from build123d import *

# Parameters (mm, degrees)
SKETCH2_W            = 120
SKETCH2_H            = 120
BOSS_EXTRUDE1_DEPTH  = 8
SKETCH4_R            = 12.5
CUT_EXTRUDE1_DEPTH   = 86.229103011
SKETCH6_R            = 5
CUT_EXTRUDE2_DEPTH   = 86.229103011
LPATTERN1_COUNT      = 2
LPATTERN1_PITCH      = 80
LPATTERN1_COUNT_DIR2 = 2
LPATTERN1_PITCH_DIR2 = 80
FILLET2_R            = 20


with BuildPart() as part:
    # Sketch2 → Boss-Extrude1 (new body)
    with BuildSketch(Plane.XY):
        Rectangle(SKETCH2_W, SKETCH2_H)
    extrude(amount=BOSS_EXTRUDE1_DEPTH)

    # Sketch4 → Cut-Extrude1 (cut, through all)
    with BuildSketch(Plane.XY.offset(8)):
        Circle(SKETCH4_R)
    extrude(amount=-CUT_EXTRUDE1_DEPTH, mode=Mode.SUBTRACT)

    # Sketch6 → Cut-Extrude2 (cut, through all)
    with BuildSketch(Plane.XY.offset(8)):
        with Locations((-40, 40)):
            Circle(SKETCH6_R)
    cut_extrude2 = extrude(amount=-CUT_EXTRUDE2_DEPTH, mode=Mode.SUBTRACT)

    # LPattern1: Cut-Extrude2 2 × 2
    with Locations(*[(i * LPATTERN1_PITCH, -j * LPATTERN1_PITCH_DIR2, 0) for i in range(LPATTERN1_COUNT) for j in range(LPATTERN1_COUNT_DIR2) if (i, j) != (0, 0)]):
        add(cut_extrude2, mode=Mode.SUBTRACT)

    # Fillet2
    fillet2_edges = [part.edges().sort_by_distance(p)[0] for p in [
        (60, -60, 4),
        (60, 60, 4),
    ]]
    fillet(fillet2_edges, radius=FILLET2_R)


solid = part.part
CAD build for the part. Positions are in the model's coordinates, mm. Give positions to 0.01 mm unless a question says otherwise; leave off trailing zeros. Loops run counter-clockwise (first coordinate to the right, second up) from the corner with the lowest first, then second, coordinate; pieces in that order, holes last. Notation, with made-up numbers: M 40.5,-36.75 L 87.5,-36.75 A16 ccw 87.5,-12.75 Z; hole C 10.5,74.5 d8. An arc over 180 degrees is marked long. Write each question's results on one line, items separated by ' | '.
Q1. Flat gauge pins, fed straight in: P1, Ø8, axis at x = 40, y = 40, coming from the +Z side; P2, Ø1.5, axis at x = 47.5, z = 1, coming from the -Y side. Where does each tip first touch, or does it go through?
Geometry check:
P1: passes through | P2: stops at y = -58.83
Q2. Mould opens along Y. For faces 1 (the face through (-14, 1, 0)), 2 (the face through (-11, -60, 4)), 3 (the face through (-45, -40, 4)) say: pulls with the +Y half, pulls with the -Y half, needs draft (parallel to the pull), parting line crosses it, or undercut.
Geometry check:
face 1: needs draft | face 2: pulls with the -Y half | face 3: undercut
Q3. Band-saw the part on B-B on z = 1.5. Write the cut outline in (x, y).
Geometry check:
outline: M -60,-60 L 40,-60 A20 ccw 60,-40 L 60,40 A20 ccw 40,60 L -60,60 Z; hole C -40,-40 d10; hole C -40,40 d10; hole C 0,0 d25; hole C 40,-40 d10; hole C 40,40 d10
Q4. Band-saw the part on A-A on y = 7.5. Write the cut outline in (x, z), and give its area (3 significant figures).
Geometry check:
outline: M -60,0 L -10,0 L -10,8 L -60,8 Z; M 10,0 L 60,0 L 60,8 L 10,8 Z | area: 800 mm²
Q5. Probe probe 1 along Y at (x, z) = (-40, 4); probe 2 along Y at (x, z) = (0, 2.75); probe 3 along X at (y, z) = (39, 4.75). List the from-to ranges inside material, lowest first.
Geometry check:
probe 1: y = -60 to -45, -35 to 35, 45 to 60 | probe 2: y = -60 to -12.5, 12.5 to 60 | probe 3: x = -60 to -44.9, -35.1 to 35.1, 44.9 to 60
Q6. Band-saw the part on C-C on x = 0. Write the cut outline in (y, z).
Geometry check:
outline: M -60,0 L -12.5,0 L -12.5,8 L -60,8 Z; M 12.5,0 L 60,0 L 60,8 L 12.5,8 Z
Q7. Band-saw the part on D-D on x = -40. Write the cut outline in (y, z).
Geometry check:
outline: M -60,0 L -45,0 L -45,8 L -60,8 Z; M -35,0 L 35,0 L 35,8 L -35,8 Z; M 45,0 L 60,0 L 60,8 L 45,8 Z
